Input: part model. Units: mm. Frame: model coordinates. Round coordinates to 2 decimals unless told otherwise and drop trailing zeros. One line per item, written item: value. Start each with the question number.
from build123d import *

# Parameters (mm, degrees)
SKETCH_1_R      = 1.5
EXTRUDE_1_DEPTH = 3
FILLET_1_R      = 3
FILLET_2_R      = 1


with BuildPart() as part:
    # 草图1 → 凸台-拉伸1 (new body)
    with BuildSketch(Plane.XY):
        with BuildLine():
            Line((-37.525, 11.5), (37.525, 11.5))
            Line((37.525, 11.5), (37.525, 4))
            ThreePointArc((37.525, 4), (37.171446609, 3.146446609), (38.025, 3.5))
            Line((38.025, 3.5), (43.525, 3.5))
            Line((43.525, 3.5), (43.525, -6.5))
            Line((43.525, -6.5), (38.025, -6.5))
            ThreePointArc((38.025, -6.5), (37.171446609, -6.146446609), (37.525, -7))
            Line((37.525, -7), (37.525, -11.5))
            Line((37.525, -11.5), (-37.525, -11.5))
            Line((-37.525, -11.5), (-37.525, -7))
            ThreePointArc((-37.525, -7), (-37.171446609, -6.146446609), (-38.025, -6.5))
            Line((-38.025, -6.5), (-43.525, -6.5))
            Line((-43.525, -6.5), (-43.525, 3.5))
            Line((-43.525, 3.5), (-38.025, 3.5))
            ThreePointArc((-38.025, 3.5), (-37.171446609, 3.146446609), (-37.525, 4))
            Line((-37.525, 4), (-37.525, 11.5))
        make_face()
        with Locations((34.525, 3.5)):
            Circle(SKETCH_1_R, mode=Mode.SUBTRACT)
        with Locations((34.525, -6.5)):
            Circle(SKETCH_1_R, mode=Mode.SUBTRACT)
        with Locations(Location((-34.525, -6.5, 0), (0, 0, 180))):
            Circle(SKETCH_1_R, mode=Mode.SUBTRACT)
        with Locations(Location((-34.525, 3.5, 0), (0, 0, 180))):
            Circle(SKETCH_1_R, mode=Mode.SUBTRACT)
    extrude(amount=EXTRUDE_1_DEPTH)

    # 圆角1
    fillet_1_edges = [part.edges().sort_by_distance(p)[0] for p in [
        (37.525, -11.5, 1.5),
        (-37.525, -11.5, 1.5),
        (-43.525, -6.5, 1.5),
        (-43.525, 3.5, 1.5),
        (-37.525, 11.5, 1.5),
        (37.525, 11.5, 1.5),
        (43.525, 3.5, 1.5),
        (43.525, -6.5, 1.5),
    ]]
    fillet(fillet_1_edges, radius=FILLET_1_R)

    # 圆角2
    fillet_2_edges = [part.edges().sort_by_distance(p)[0] for p in [
        (-37.525, -7, 1.5),
        (-38.025, -6.5, 1.5),
        (-38.025, 3.5, 1.5),
        (-37.525, 4, 1.5),
        (37.525, 4, 1.5),
        (38.025, 3.5, 1.5),
        (38.025, -6.5, 1.5),
        (37.525, -7, 1.5),
    ]]
    fillet(fillet_2_edges, radius=FILLET_2_R)


solid = part.part
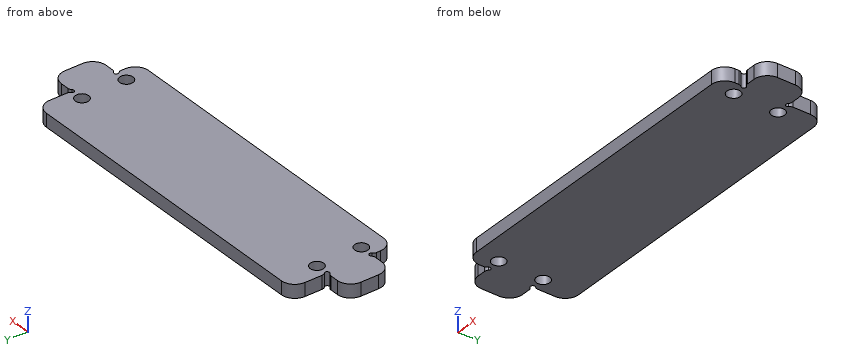
Item 1: Section query A-A on z = 1.4. Give the number of separate pieces and of enclosed holes in the cut face, and give its area (3 significant figures).
Item 2: Line query: L1, parallel to X at y = 2.5, z = 1.5; L2, parallel to X at y = 7.25, z = 2.75 (3 decimals); L3, parallel to X at y = -10.25, z = 0.45. Output: solid intervals per line, ascending.
Item 3: First-contact query: pin 1 Ø1.8 at (x, y) = (34.525, 3.5) entering from +Z; pin 2 Ø4 at (x, y) = (34.525, -6.5) entering from +Z; pin 3 Ø0.9 at (x, z) = (39, 1.5) entering from +Y. Flat tips, straight axial feed; report the tip coordinate or a pass-through.
Geometry results:
1. separate pieces: 1
1. enclosed holes: 4
1. area: 1,800 mm^2
2. L1: x = -42.76 to -35.64, -33.41 to 33.41, 35.64 to 42.76
2. L2: x = -37.525 to 37.525
2. L3: x = -36.96 to 36.96
3. pin 1: passes through
3. pin 2: stops at z = 3
3. pin 3: stops at y = 3.5
